Read the model definition and answer for the solid it produces. Units are mm, in the model's axes. Coordinates: 2 decimals unless noted, no trailing zeros. Write each loop counter-clockwise with the first axis right and the second up, starting at its lowest first coordinate (ties: lowest second). Pieces come first, ordered by that corner, then holes.
1) Find the intervals of material crossed by line 1 (X direction, y = 12.5, z = 841.5), in increasing order.
2) The part is cut by section A-A (z = 228.5). Determine the outline of the cut face in (x, y).
3) The part is cut by section B-B (y = 7). Determine the outline of the cut face in (x, z), then the cut area to 3 significant figures.
4) Each of these flat-tipped pins is pushed along its axis until it touches: pin 1 Ø3 at (y, z) = (15, 123) entering from +X; pin 2 Ø11 at (x, z) = (1.5, 428.5) entering from +Y. Where does it stop, or does it pass through?
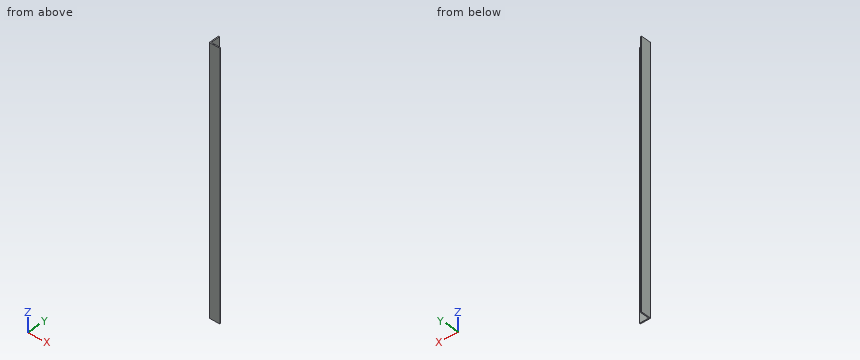
Autodesk Inventor part; units mm, degrees
ref_plane "YZ Plane" through (0, 0, 0) normal (1, 0, 0) x (0, 1, 0)
ref_plane "XZ Plane" through (0, 0, 0) normal (0, 1, 0) x (-1, 0, 0)
ref_plane "XY Plane" through (0, 0, 0) normal (0, 0, 1) x (1, 0, 0)
sketch "Boceto1" plane through (0, 0, 0) normal (0, 0, 1) x (1, 0, 0)
  line L0 (-20, 20) -> (20, 20)
  line L1 (20, 20) -> (20, -20)
  line L2 (20, -20) -> (-20, -20)
  line L3 (-20, -20) -> (-20, 20)
  line L4 (-20, 20) -> (20, -20) construction
  line L5 (-16, 16) -> (16, 16)
  line L6 (16, 16) -> (16, -16)
  line L7 (16, -16) -> (-16, -16)
  line L8 (-16, -16) -> (-16, 16)
  line L9 (-16, 0) -> (-20, 0) construction
  line L10 (0, 16) -> (0, 20) construction
  line L11 (16, 0) -> (20, 0) construction
  line L12 (0, -16) -> (0, -20) construction
  line L13 (-16, 16) -> (-16, 20)
  line L14 (16, -16) -> (20, -16)
  point P0 (0, 0)
  point P1 (0, 0)
  dimension "d0" = 40
  dimension "d1" = 4
  dimension "d4" = 40
extrude "Extrusión1" add sketch "Boceto1" along normal blind 992 contours L0 L13 L8 L7 L14 L1 L2 L3
properties part number "C_358_40_2"
Reported:
1. line 1: x = -20 to -16
2. outline: (-20, -20) - (20, -20) - (20, -16) - (-16, -16) - (-16, 20) - (-20, 20) - close
3. outline: (-20, 0) - (-16, 0) - (-16, 992) - (-20, 992) - close
3. area: 3,970 mm2
4. pin 1: stops at x = -16
4. pin 2: stops at y = -16
